```python
from build123d import *

# Parameters (mm, degrees)
BOSS_EXTRUDE1_DEPTH = 170
FILLET1_R           = 2
FILLET2_R           = 2
SKETCH2_R           = 5
CUT_EXTRUDE2_DEPTH  = 455


with BuildPart() as part:
    # Sketch1 → Boss-Extrude1 (new body)
    with BuildSketch(Plane.XY):
        Polygon((-43.543195893, -41.265832091), (-43.543195893, 35.734167909), (-46.543195893, 35.734167909), (-46.543195893, -44.265832091), (133.456804107, -44.265832091), (133.456804107, 35.734167909), (130.456804107, 35.734167909), (130.456804107, -41.265832091), align=None)
    extrude(amount=BOSS_EXTRUDE1_DEPTH)

    # Fillet1
    fillet1_edges = [part.edges().sort_by_distance(p)[0] for p in [
        (-46.543195893, -44.265832091, 85),
    ]]
    fillet(fillet1_edges, radius=FILLET1_R)

    # Fillet2
    fillet2_edges = [part.edges().sort_by_distance(p)[0] for p in [
        (133.456804107, -44.265832091, 85),
    ]]
    fillet(fillet2_edges, radius=FILLET2_R)

    # Sketch2 → Cut-Extrude2 (cut)
    with BuildSketch(Plane(origin=(133.456804107, 0, 0), x_dir=(0, 0, -1), z_dir=(1, 0, 0))):
        with Locations((-150, -3.265832091)):
            Circle(SKETCH2_R)
        with Locations((-20, -3.265832091)):
            Circle(SKETCH2_R)
    extrude(amount=-CUT_EXTRUDE2_DEPTH, mode=Mode.SUBTRACT)


solid = part.part
```
Could you check a few things on this model? Use its own coordinates, in mm. A direction names the side the tool comes from. Give positions to 0.01 mm unless a question says otherwise; leave off trailing zeros. Loops run counter-clockwise (first coordinate to the right, second up) from the corner with the lowest first, then second, coordinate; pieces in that order, holes last. Notation, with made-up numbers: (-31, 31) -> (-8, 31) arc R22 cw to (-8, 51) -> close; hole circle Ø4 at (24.25, 49). An arc over 180 degrees is marked (long way). Put each result on its own line as item: value.
(1) Imagine slicing it at D-D on x = 81. Write out the boundary of the cut face in (y, z).
Computed:
outline: (-44.27, 0) -> (-41.27, 0) -> (-41.27, 170) -> (-44.27, 170) -> close
(2) Thinking about a two-plate mould opening in Z: for faces 1 (the face through (42, -44.266, 84)), 2 (the face through (3, -43, 0)), 3 (the face through (131.978, -3.046, 154.995)), 4 (the face through (-45.022, -3.046, 24.995)), which applies, pulls with the +Z half, pulls with the -Z half, needs draft (parallel to the pull), parting line crosses it, or undercut?
Computed:
face 1: needs draft
face 2: pulls with the -Z half
face 3: undercut
face 4: undercut
(3) For faces 5 (the face through (130.457, -2, 84)), 6 (the face through (-45.022, -3.046, 154.995)), which set-ups out of +Z, -Z, +X, -X, +Y, -Y let a thin tool reach every point of the face, with its end or its side?
Computed:
face 5: +Z, -Z, +Y
face 6: +X, -X
(4) Imagine slicing it at B-B on y = -18.5. Write out the boundary of the cut face in (x, z).
Computed:
outline: (-46.54, 0) -> (-43.54, 0) -> (-43.54, 170) -> (-46.54, 170) -> close; (130.46, 0) -> (133.46, 0) -> (133.46, 170) -> (130.46, 170) -> close
(5) Please list where these lines run through material, in increasing order: probe 1 along Y at (x, z) = (-44.65, 150); probe 2 along X at (y, z) = (-10, 148.5); probe 3 along Y at (x, z) = (98, 19). Write a range as [from, to].
Computed:
probe 1: [-44.26, -8.27], [1.73, 35.73]
probe 2: [-46.54, -43.54], [130.46, 133.46]
probe 3: [-44.27, -41.27]
(6) I'm going to push flat-ended pins straight in: pin 1 Ø12 at (x, z) = (6, 53) entering from +Y; pin 2 Ø9 at (y, z) = (-3.27, 20) entering from +X. Where does each tip first touch, or does it pass through?
Computed:
pin 1: y = -41.27
pin 2: through
(7) Imagine slicing it at A-A on z = 20. Write out the boundary of the cut face in (x, y).
Computed:
outline: (-46.54, -42.27) arc R2 ccw to (-44.54, -44.27) -> (131.46, -44.27) arc R2 ccw to (133.46, -42.27) -> (133.46, -8.27) -> (130.46, -8.27) -> (130.46, -41.27) -> (-43.54, -41.27) -> (-43.54, -8.27) -> (-46.54, -8.27) -> close; (-46.54, 1.73) -> (-43.54, 1.73) -> (-43.54, 35.73) -> (-46.54, 35.73) -> close; (130.46, 1.73) -> (133.46, 1.73) -> (133.46, 35.73) -> (130.46, 35.73) -> close
(8) Imagine slicing it at C-C on z = 85.5. Write out the boundary of the cut face in (x, y), plus the area to 3 significant figures.
Computed:
outline: (-46.54, -42.27) arc R2 ccw to (-44.54, -44.27) -> (131.46, -44.27) arc R2 ccw to (133.46, -42.27) -> (133.46, 35.73) -> (130.46, 35.73) -> (130.46, -41.27) -> (-43.54, -41.27) -> (-43.54, 35.73) -> (-46.54, 35.73) -> close
area: 1,000 mm^2
